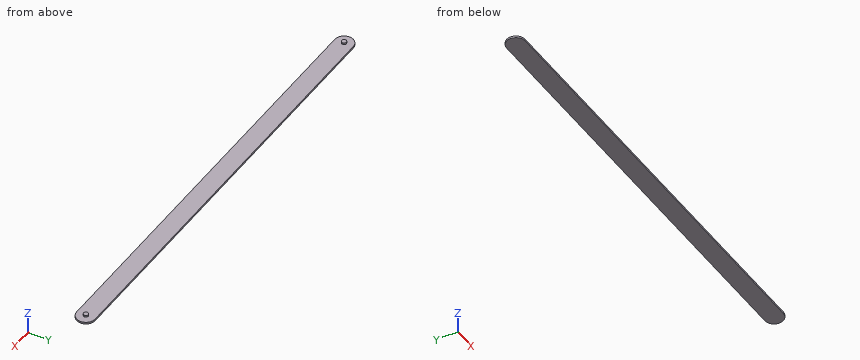
```python
from build123d import *

# Parameters (mm, degrees)
BOSS_EXTRUDE1_DEPTH = 2.54
BOSS_EXTRUDE2_DEPTH = 5.08


with BuildPart() as part:
    # Sketch2 → Boss-Extrude1 (new body)
    with BuildSketch(Plane.XY):
        with BuildLine():
            ThreePointArc((12.7, 12.7), (8.980256121, 3.719743879), (0, 0))
            Line((0, 0), (584.2, 0))
            ThreePointArc((584.2, 0), (571.5, 12.7), (584.2, 25.4))
            Line((584.2, 25.4), (0, 25.4))
            ThreePointArc((0, 25.4), (8.980256121, 21.680256121), (12.7, 12.7))
        make_face()
        with BuildLine():
            ThreePointArc((584.2, 25.4), (571.5, 12.7), (584.2, 0))
            Line((584.2, 0), (584.2, 9.525))
            ThreePointArc((584.2, 9.525), (581.025, 12.7), (584.2, 15.875))
            Line((584.2, 15.875), (584.2, 25.4))
        make_face()
        with BuildLine():
            Line((584.2, 9.525), (584.2, 0))
            ThreePointArc((584.2, 0), (593.180256121, 3.719743879), (596.9, 12.7))
            ThreePointArc((596.9, 12.7), (593.180256121, 21.680256121), (584.2, 25.4))
            Line((584.2, 25.4), (584.2, 15.875))
            ThreePointArc((584.2, 15.875), (586.44506403, 14.94506403), (587.375, 12.7))
            ThreePointArc((587.375, 12.7), (586.44506403, 10.45493597), (584.2, 9.525))
        make_face()
        with BuildLine():
            ThreePointArc((0, 25.4), (-12.7, 12.7), (0, 0))
            Line((0, 0), (0, 9.525))
            ThreePointArc((0, 9.525), (-3.175, 12.7), (0, 15.875))
            Line((0, 15.875), (0, 25.4))
        make_face()
        with BuildLine():
            Line((0, 9.525), (0, 0))
            ThreePointArc((0, 0), (8.980256121, 3.719743879), (12.7, 12.7))
            ThreePointArc((12.7, 12.7), (8.980256121, 21.680256121), (0, 25.4))
            Line((0, 25.4), (0, 15.875))
            ThreePointArc((0, 15.875), (2.24506403, 14.94506403), (3.175, 12.7))
            ThreePointArc((3.175, 12.7), (2.24506403, 10.45493597), (0, 9.525))
        make_face()
    extrude(amount=BOSS_EXTRUDE1_DEPTH)

    # Sketch2_3 → Boss-Extrude2 (add)
    with BuildSketch(Plane.XY):
        with BuildLine():
            ThreePointArc((0, 15.875), (-3.175, 12.7), (0, 9.525))
            Line((0, 9.525), (0, 15.875))
        make_face()
        with BuildLine():
            Line((0, 15.875), (0, 9.525))
            ThreePointArc((0, 9.525), (2.24506403, 10.45493597), (3.175, 12.7))
            ThreePointArc((3.175, 12.7), (2.24506403, 14.94506403), (0, 15.875))
        make_face()
        with BuildLine():
            ThreePointArc((584.2, 15.875), (581.025, 12.7), (584.2, 9.525))
            Line((584.2, 9.525), (584.2, 15.875))
        make_face()
        with BuildLine():
            Line((584.2, 15.875), (584.2, 9.525))
            ThreePointArc((584.2, 9.525), (586.44506403, 10.45493597), (587.375, 12.7))
            ThreePointArc((587.375, 12.7), (586.44506403, 14.94506403), (584.2, 15.875))
        make_face()
    extrude(amount=BOSS_EXTRUDE2_DEPTH)


solid = part.part
```
Build history of the part. All positions in model axes, mm. Give positions to 0.01 mm unless a question says otherwise; leave off trailing zeros. Loops run counter-clockwise (first coordinate to the right, second up) from the corner with the lowest first, then second, coordinate; pieces in that order, holes last. Notation, with made-up numbers: (46, 68) -> (59, 68) arc R25 ccw to (59, 90) -> close; hole circle Ø6 at (43.25, 4). An arc over 180 degrees is marked (long way). One line per question, with ' | ' between items.
Q1. Drop a flat-ended pin along its axis: pin 1 (12.5 mm diameter, centred on x = 444.5, y = 7, fed in from +Z). Give the stop position or say it passes through.
Filled sheet:
pin 1: stops at z = 2.54
Q2. Drill centre lines: line 1 along X through (y, z) = (13.75, 1.05); line 2 along Z through (x, y) = (50.5, 8.5); line 3 along X through (y, z) = (15.25, 3.1). Where is each one in solid material? Low to high. Write a range as [from, to].
Filled sheet:
line 1: x = [-12.66, 596.86] | line 2: z = [0, 2.54] | line 3: x = [-1.89, 1.89], [582.31, 586.09]
Q3. Cut at B-B, the plane x = 536. Write the cut outline in (y, z).
Filled sheet:
outline: (0, 0) -> (25.4, 0) -> (25.4, 2.54) -> (0, 2.54) -> close
Q4. Cut at A-A, the plane z = 4.3. Write the cut outline in (x, y) (3 decimals).
Filled sheet:
outline: circle Ø6.35 at (0, 12.7); circle Ø6.35 at (584.2, 12.7)
Q5. Cut at C-C, the plane y = 5.5. Write the cut outline in (x, z).
Filled sheet:
outline: (-10.46, 0) -> (594.66, 0) -> (594.66, 2.54) -> (-10.46, 2.54) -> close
